Geometry check sheet. Reference: drawing and pictorial views, mm from the part's lowest x, y, z. Give positions to 0.01 mm unless a question says otherwise; leave off trailing zeros. Order: outer loops, then holes, each group sorted by start corner. A loop starts at its lowest first (then second) coordinate and runs counter-clockwise, first axis right, second up. Notation, with made-up numbers: M -2,0 L 2,0 A35 ccw 2,38 Z; hole C 69,-39.75 d4. An arc over 180 degrees is marked long. Answer as a JSON object with one key per item and string values. Group by question number.
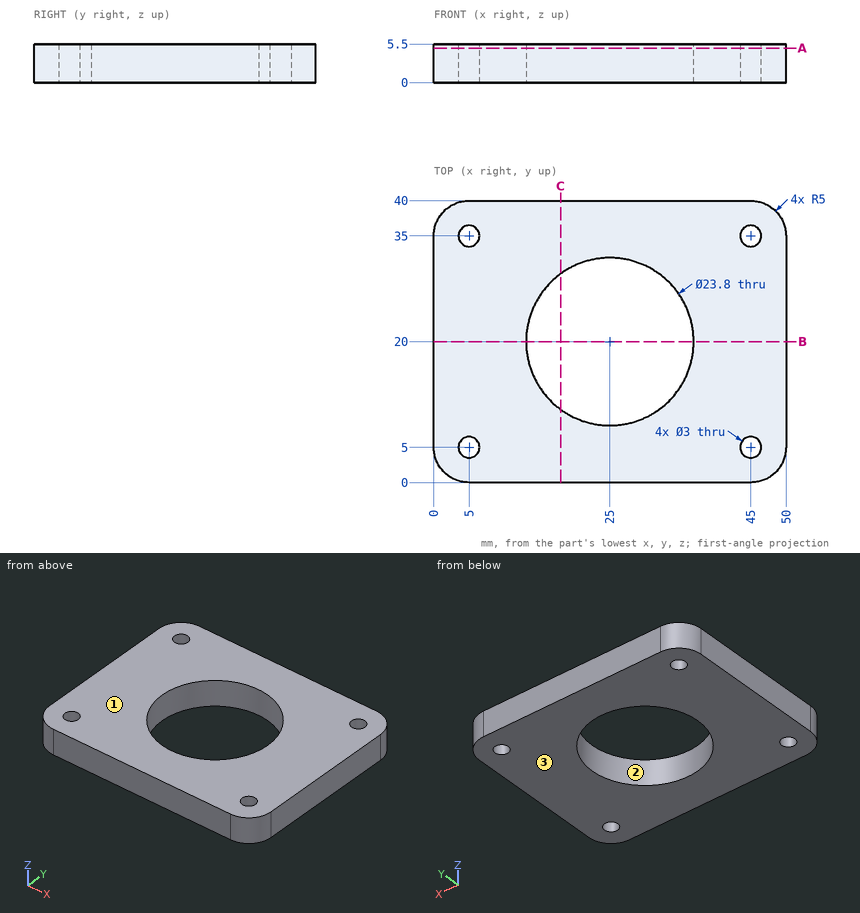
1. Depth check by flat-ended pin: pin 1 (1 mm diameter, centred on x = 38.5, z = 3, fed in from -Y); pin 2 (14.5 mm diameter, centred on x = 25, y = 20, fed in from +Z). Enter the tip coordinate at first touch or a pass-through.
2. Thickness scan on line 1 along Y through (x, z) = (45, 4.25); line 2 along X through (y, z) = (4, 4.3); line 3 along X through (y, z) = (35.5, 4.85). Record the ranges inside material, lowest first. Write a range as [from, to].
3. Cross-section at A-A (z = 4.9). Record the cut outline in (x, y), and give its area (3 significant figures).
4. Release check for a two-part mould opening along Z. For the marked faces 1, 2 and 3 record: released by +Z, released by -Z, zero draft, split by the parting line, or undercut.
5. Cross-section at C-C (x = 18). Record the cut outline in (y, z), and give its area (3 significant figures).
6. Cross-section at B-B (y = 20). Record the cut outline in (x, z).
Report:
{
 "1": {"pin 1": "stops at y = 0", "pin 2": "passes through"},
 "2": {"line 1": "y = [0, 3.5], [6.5, 33.5], [36.5, 40]", "line 2": "x = [0.1, 3.88], [6.12, 43.88], [46.12, 49.9]", "line 3": "x = [0.03, 3.59], [6.41, 43.59], [46.41, 49.97]"},
 "3": {"outline": "M 0,5 A5 ccw 5,0 L 45,0 A5 ccw 50,5 L 50,35 A5 ccw 45,40 L 5,40 A5 ccw 0,35 Z; hole C 5,5 d3; hole C 5,35 d3; hole C 25,20 d23.8; hole C 45,5 d3; hole C 45,35 d3", "area": "1,510 mm2"},
 "4": {"face 1": "released by +Z", "face 2": "zero draft", "face 3": "released by -Z"},
 "5": {"outline": "M 0,0 L 10.38,0 L 10.38,5.5 L 0,5.5 Z; M 29.62,0 L 40,0 L 40,5.5 L 29.62,5.5 Z", "area": "114 mm2"},
 "6": {"outline": "M 0,0 L 13.1,0 L 13.1,5.5 L 0,5.5 Z; M 36.9,0 L 50,0 L 50,5.5 L 36.9,5.5 Z"}
}
